from build123d import *

# Parameters (mm, degrees)
SKETCH1_R           = 3.5
BOSS_EXTRUDE1_DEPTH = 5
FILLET1_R           = 1
FILLET2_R           = 1
FILLET3_R           = 1
FILLET4_R           = 1


with BuildPart() as part:
    # Sketch1 → Boss-Extrude1 (new body)
    with BuildSketch(Plane.XY):
        with BuildLine():
            Line((0, 0), (-100, 0))
            Line((-100, 0), (-100, -80))
            Line((-100, -80), (-100, -83))
            ThreePointArc((-100, -83), (-97.949747468, -87.949747468), (-93, -90))
            Line((-93, -90), (-92, -90))
            Line((-92, -90), (-65, -90))
            Line((-65, -90), (-65, -78.819347292))
            ThreePointArc((-65, -78.819347292), (-50, -25), (-35, -78.819347292))
            Line((-35, -78.819347292), (-35, -90))
            Line((-35, -90), (-8, -90))
            Line((-8, -90), (-7, -90))
            ThreePointArc((-7, -90), (-2.050252532, -87.949747468), (0, -83))
            Line((0, -83), (0, -80))
            Line((0, -80), (0, 0))
        make_face()
        with Locations((-50, -16.5)):
            Circle(SKETCH1_R, mode=Mode.SUBTRACT)
        with Locations((-12, -54)):
            Circle(SKETCH1_R, mode=Mode.SUBTRACT)
        with Locations((-17, -74)):
            Circle(SKETCH1_R, mode=Mode.SUBTRACT)
        with Locations((-18, -35)):
            Circle(SKETCH1_R, mode=Mode.SUBTRACT)
        with Locations(Location((-83, -74, 0), (0, 0, 180))):
            Circle(SKETCH1_R, mode=Mode.SUBTRACT)
        with Locations(Location((-88, -54, 0), (0, 0, 180))):
            Circle(SKETCH1_R, mode=Mode.SUBTRACT)
    extrude(amount=BOSS_EXTRUDE1_DEPTH)

    # Fillet1
    fillet1_edges = [part.edges().sort_by_distance(p)[0] for p in [
        (-100, 0, 2.5),
    ]]
    fillet(fillet1_edges, radius=FILLET1_R)

    # Fillet2
    fillet2_edges = [part.edges().sort_by_distance(p)[0] for p in [
        (0, 0, 2.5),
    ]]
    fillet(fillet2_edges, radius=FILLET2_R)

    # Fillet3
    fillet3_edges = [part.edges().sort_by_distance(p)[0] for p in [
        (-65, -90, 2.5),
    ]]
    fillet(fillet3_edges, radius=FILLET3_R)

    # Fillet4
    fillet4_edges = [part.edges().sort_by_distance(p)[0] for p in [
        (-35, -90, 2.5),
    ]]
    fillet(fillet4_edges, radius=FILLET4_R)


solid = part.part
Source: CAD feature listing. Evaluate the final solid. Frame: model axes, mm. A direction names the side the tool comes from. Coordinates: 2 decimals unless noted, no trailing zeros. Loops run counter-clockwise (first coordinate to the right, second up) from the corner with the lowest first, then second, coordinate; pieces in that order, holes last. Notation, with made-up numbers: (47.25, -9.5) - (82.25, -9.5) arc R25 cw to (82.25, 20.5) - close; hole circle Ø5 at (41.5, 40). An arc over 180 degrees is marked (long way). One line per question, with ' | ' between items.
1) Pull-direction query (X, two-part tool) for faces 3 (the face through (-15.385, -77.105, 2.465)), 4 (the face through (-51, -24, 5)), 5 (the face through (-100, -41, 2)); classes: released by +X, released by -X, zero draft, split by the parting line, or undercut.
Report:
face 3: undercut | face 4: zero draft | face 5: released by -X
2) Line query: line 1 along Y through (x, z) = (-12, 3.05); line 2 along X through (y, z) = (-78.5, 3.2); line 3 along Y through (x, z) = (-74, 0.4). Output: solid intervals per line, ascending.
Report:
line 1: y = -90 to -57.5, -50.5 to 0 | line 2: x = -100 to -65.52, -34.48 to 0 | line 3: y = -90 to -70.28, -37.72 to 0
3) Set-up query: faces 1 (the face through (-98, -87.9, 2.5)), 2 (the face through (-65, -84, 2)). Return all of +Z, -Z, +X, -X, +Y, -Y with unobstructed straight access to the full face (end or side cutting, diameter ignored); none if empty.
Report:
face 1: +Z, -Z, -X, -Y | face 2: +Z, -Z, -Y
4) Section B-B, the plane x = -88. Return loops of the section in (y, z), then the cut area to 3 significant figures.
Report:
outline: (-90, 0) - (-57.5, 0) - (-57.5, 5) - (-90, 5) - close; (-50.5, 0) - (0, 0) - (0, 5) - (-50.5, 5) - close | area: 415 mm²
5) Section D-D, the plane z = 0.8. Return loops of the section in (x, y), then the cut area to 3 significant figures.
Report:
outline: (-100, -83) arc R7 ccw to (-93, -90) - (-66, -90) arc R1 ccw to (-65, -89) - (-65, -78.82) arc R29 cw (long way) to (-35, -78.82) - (-35, -89) arc R1 ccw to (-34, -90) - (-7, -90) arc R7 ccw to (0, -83) - (0, -1) arc R1 ccw to (-1, 0) - (-99, 0) arc R1 ccw to (-100, -1) - close; hole circle Ø7 at (-88, -54); hole circle Ø7 at (-83, -74); hole circle Ø7 at (-50, -16.5); hole circle Ø7 at (-18, -35); hole circle Ø7 at (-17, -74); hole circle Ø7 at (-12, -54) | area: 5,850 mm²
6) Section C-C, the plane y = -16.5. Return loops of the section in (x, z), then the cut area to 3 significant figures.
Report:
outline: (-100, 0) - (-53.5, 0) - (-53.5, 5) - (-100, 5) - close; (-46.5, 0) - (0, 0) - (0, 5) - (-46.5, 5) - close | area: 465 mm²
7) First-contact query: P1, Ø1.5, axis at y = -84, z = 2.5, coming from the +X side. Flat tip, straight axial feed; report the tip coordinate or a pass-through.
Report:
P1: stops at x = 0
8) Section A-A, the plane y = -74. Return loops of the section in (x, z).
Report:
outline: (-100, 0) - (-86.5, 0) - (-86.5, 5) - (-100, 5) - close; (-79.5, 0) - (-71, 0) - (-71, 5) - (-79.5, 5) - close; (-29, 0) - (-20.5, 0) - (-20.5, 5) - (-29, 5) - close; (-13.5, 0) - (0, 0) - (0, 5) - (-13.5, 5) - close
